Check sheet for the drawn part. Datum: minimum x, y, z corner. Units: mm. A direction names the side the tool comes from. Round coordinates to 2 decimals unless told otherwise and drop trailing zeros. Write each loop counter-clockwise with the first axis right and the second up, starting at its lowest first coordinate (ties: lowest second). Pieces come first, ordered by that corner, then holes. Notation, with made-up numbers: M -37,-3.5 L -5,-3.5 A11 cw -5,17.5 Z; hole C 83,57.25 d1. An arc over 180 degrees is marked long. One line per item, written item: value.
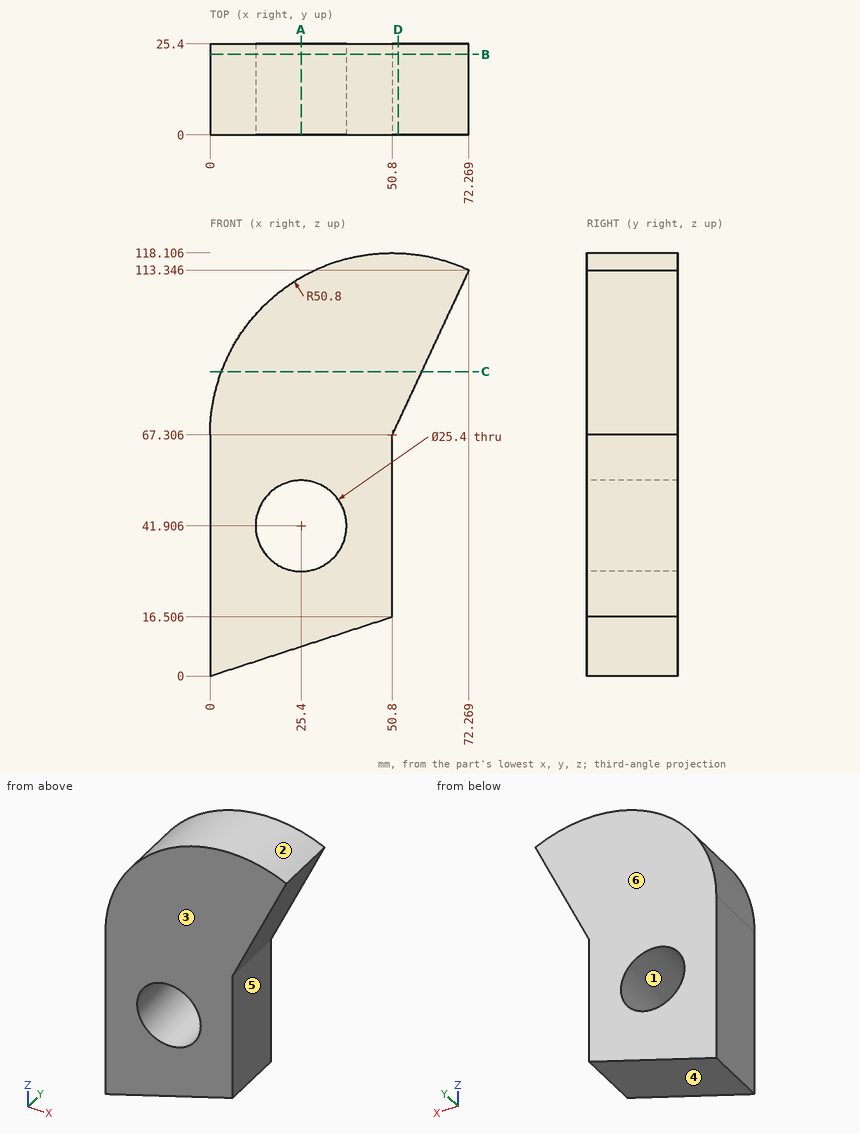
Q1. Sectioned sample at C-C on z = 85. Enter the section's corners in (x, y), and give its area (3 significant figures).
Completed:
outline: M 3.18,0 L 59.05,0 L 59.05,25.4 L 3.18,25.4 Z
area: 1,420 mm^2
Q2. Depth check by flat-ended pin: P1, Ø5, axis at y = 15, z = 82, coming from the -X side (1 decimal); P2, Ø12, axis at y = 15.5, z = 77, coming from the -X side; P3, Ø10, axis at x = 61, y = 4, coming from the +Z side. Enter the tip coordinate at first touch or a pass-through.
Completed:
P1: x = 1.5
P2: x = 0.13
P3: z = 117.84
Q3. Sectioned sample at A-A on x = 25.4. Enter the section's corners in (y, z), and give its area (3 significant figures).
Completed:
outline: M 0,8.25 L 25.4,8.25 L 25.4,29.21 L 0,29.21 Z; M 0,54.61 L 25.4,54.61 L 25.4,111.3 L 0,111.3 Z
area: 1,970 mm^2
Q4. Draft check along X on the marked faces 1, 2, 3 and 4. Enter one of: pulls with the +X half, pulls with the -X half, needs draft (parallel to the pull), parting line crosses it, or undercut.
Completed:
face 1: undercut
face 2: parting line crosses it
face 3: needs draft
face 4: pulls with the +X half
Q5. Scan lines: line 1 (X direction, y = 4, z = 41.5); line 2 (X direction, y = 20.25, z = 23); line 3 (Z direction, x = 25.4, y = 10.75) (1 decimal). Record each from-to range of solid material in increasing order. Write a range as [from, to].
Completed:
line 1: [0, 12.71], [38.09, 50.8]
line 2: [0, 50.8]
line 3: [8.3, 29.2], [54.6, 111.3]
Q6. Sectioned sample at D-D on x = 52.5. Enter the section's corners in (y, z), and give its area (3 significant figures).
Completed:
outline: M 0,70.95 L 25.4,70.95 L 25.4,118.08 L 0,118.08 Z
area: 1,200 mm^2
Q7. Sectioned sample at B-B on y = 22.5. Enter the section's corners in (x, z), and give its area (3 significant figures).
Completed:
outline: M 0,0 L 50.8,16.51 L 50.8,67.31 L 72.27,113.35 A50.8 ccw 0,67.31 Z; hole C 25.4,41.91 d25.4
area: 5,080 mm^2
Q8. Access from +Z, -Z, +X, -X, +Y, -Y to the whole of each face (thin tool, end or side, straight path). Record for the marked faces 5 and 6.
Completed:
face 5: -Z, +X, +Y, -Y
face 6: +Z, -Z, +X, -X, +Y
